```python
from build123d import *

# Parameters (mm, degrees)
BOSS_EXTRUDE1_DEPTH          = 5
BOSS_EXTRUDE1_DEPTH_BACK     = 7.5
SKETCH2_W                    = 57.31
SKETCH2_H                    = 43.46
SKETCH2_W_2                  = 53.31
SKETCH2_H_2                  = 39.46
FILLET1_R                    = 5
SKETCH3_R                    = 1
BOSS_EXTRUDE2_DEPTH          = 3
CUT_EXTRUDE1_DEPTH           = 2
CUT_EXTRUDE1_DRAFT           = 3
SKETCH5_R                    = 1
CUT_EXTRUDE1_PROFILE_2_DEPTH = 2
CUT_EXTRUDE1_PROFILE_2_DRAFT = 3
CUT_EXTRUDE1_PROFILE_3_DEPTH = 2
CUT_EXTRUDE1_PROFILE_3_DRAFT = 3
FILLET2_R                    = 1
SKETCH6_W                    = 2
SKETCH6_H                    = 40
BOSS_EXTRUDE3_DEPTH          = 2
FILLET3_R                    = 1


with BuildPart() as part:
    # Sketch2 → Boss-Extrude1 (new, two sides: drawn at the far end of the back side and taken through both)
    with BuildSketch(Plane(origin=(0, 0, 0), x_dir=(1, 0, 0), z_dir=(0, 1, 0)).offset(-BOSS_EXTRUDE1_DEPTH_BACK)):
        with Locations((-3, -1.5)):
            Rectangle(SKETCH2_W, SKETCH2_H)
        with Locations((-3, -1.5)):
            Rectangle(SKETCH2_W_2, SKETCH2_H_2, mode=Mode.SUBTRACT)
    extrude(amount=BOSS_EXTRUDE1_DEPTH + BOSS_EXTRUDE1_DEPTH_BACK)

    # Fillet1
    fillet1_edges = [part.edges().sort_by_distance(p)[0] for p in [
        (-29.655, -1.25, 21.23),
        (-29.655, -1.25, -18.23),
        (23.655, -1.25, -18.23),
        (23.655, -1.25, 21.23),
        (-31.655, -1.25, -20.23),
        (25.655, -1.25, -20.23),
        (25.655, -1.25, 23.23),
        (-31.655, -1.25, 23.23),
    ]]
    fillet(fillet1_edges, radius=FILLET1_R)

    # Sketch3 → Boss-Extrude2 (add)
    with BuildSketch(Plane.XZ.offset(7.5)):
        with BuildLine():
            Line((-31.655, 18.23), (-31.655, -15.23))
            ThreePointArc((-31.655, -15.23), (-30.190533906, -18.765533906), (-26.655, -20.23))
            Line((-26.655, -20.23), (20.655, -20.23))
            ThreePointArc((20.655, -20.23), (24.190533906, -18.765533906), (25.655, -15.23))
            Line((25.655, -15.23), (25.655, 18.23))
            ThreePointArc((25.655, 18.23), (24.190533906, 21.765533906), (20.655, 23.23))
            Line((20.655, 23.23), (-26.655, 23.23))
            ThreePointArc((-26.655, 23.23), (-30.190533906, 21.765533906), (-31.655, 18.23))
        make_face()
        with Locations(Location((-18.155, 11.5, 0), (0, 0, 270))):
            Circle(SKETCH3_R, mode=Mode.SUBTRACT)
        with Locations(Location((17.845, 11.5, 0), (0, 0, 270))):
            Circle(SKETCH3_R, mode=Mode.SUBTRACT)
        with Locations(Location((17.845, -12.5, 0), (0, 0, 270))):
            Circle(SKETCH3_R, mode=Mode.SUBTRACT)
    extrude(amount=BOSS_EXTRUDE2_DEPTH)


with BuildPart() as cut_extrude1_tool:
    # Sketch5 → Cut-Extrude1 (with draft: the straight prism first)
    with BuildSketch(Plane.XZ.offset(10.5)):
        Polygon((-18.155, 13.924871131), (-20.255, 12.712435565), (-20.255, 10.287564435), (-18.155, 9.075128869), (-16.055, 10.287564435), (-16.055, 12.712435565), align=None)
    extrude(amount=-CUT_EXTRUDE1_DEPTH)
    # Cut-Extrude1: the draft: its side faces are tilted about the plane it starts from
    cut_extrude1_sides = [cut_extrude1_tool.faces().sort_by_distance(p)[0] for p in [
        (-19.205, -9.5, 13.318653348),
        (-20.255, -9.5, 11.5),
        (-19.205, -9.5, 9.681346652),
        (-17.105, -9.5, 9.681346652),
        (-16.055, -9.5, 11.5),
        (-17.105, -9.5, 13.318653348),
    ]]
    draft(cut_extrude1_sides, Plane.XZ.offset(10.5), CUT_EXTRUDE1_DRAFT)


with BuildPart() as part_1:
    add(part.part)

    # Cut-Extrude1: cut by cut_extrude1_tool
    add(cut_extrude1_tool.part, mode=Mode.SUBTRACT)


with BuildPart() as cut_extrude1_profile_2_tool:
    # Sketch5 → Cut-Extrude1 profile 2 (with draft: the straight prism first)
    with BuildSketch(Plane.XZ.offset(10.5)):
        Polygon((17.857823878, 13.905392128), (15.745, 12.685552694), (15.745, 10.275489302), (17.857823878, 9.055649867), (19.945, 10.260681563), (19.945, 12.700360432), align=None)
        with Locations(Location((17.845, 11.5, 0), (0, 0, 270))):
            Circle(SKETCH5_R, mode=Mode.SUBTRACT)
    extrude(amount=-CUT_EXTRUDE1_PROFILE_2_DEPTH)
    # Cut-Extrude1 profile 2: the draft: its side faces are tilted about the plane it starts from
    cut_extrude1_profile_2_sides = [cut_extrude1_profile_2_tool.faces().sort_by_distance(p)[0] for p in [
        (16.801411939, -9.5, 13.295472411),
        (15.745, -9.5, 11.480520998),
        (16.801411939, -9.5, 9.665569584),
        (18.901411939, -9.5, 9.658165715),
        (19.945, -9.5, 11.480520998),
        (18.901411939, -9.5, 13.30287628),
        (17.845, -9.5, 12.5),
    ]]
    draft(cut_extrude1_profile_2_sides, Plane.XZ.offset(10.5), CUT_EXTRUDE1_PROFILE_2_DRAFT)


with BuildPart() as part_2:
    add(part_1.part)

    # Cut-Extrude1 profile 2: cut by cut_extrude1_profile_2_tool
    add(cut_extrude1_profile_2_tool.part, mode=Mode.SUBTRACT)


with BuildPart() as cut_extrude1_profile_3_tool:
    # Sketch5 → Cut-Extrude1 profile 3 (with draft: the straight prism first)
    with BuildSketch(Plane.XZ.offset(10.5)):
        Polygon((17.833837254, -10.086917044), (15.733837254, -11.299352609), (15.733837254, -13.724223739), (17.833837254, -14.936659305), (19.933837254, -13.724223739), (19.933837254, -11.299352609), align=None)
        with Locations(Location((17.845, -12.5, 0), (0, 0, 270))):
            Circle(SKETCH5_R, mode=Mode.SUBTRACT)
    extrude(amount=-CUT_EXTRUDE1_PROFILE_3_DEPTH)
    # Cut-Extrude1 profile 3: the draft: its side faces are tilted about the plane it starts from
    cut_extrude1_profile_3_sides = [cut_extrude1_profile_3_tool.faces().sort_by_distance(p)[0] for p in [
        (16.783837254, -9.5, -10.693134826),
        (15.733837254, -9.5, -12.511788174),
        (16.783837254, -9.5, -14.330441522),
        (18.883837254, -9.5, -14.330441522),
        (19.933837254, -9.5, -12.511788174),
        (18.883837254, -9.5, -10.693134826),
        (17.845, -9.5, -11.5),
    ]]
    draft(cut_extrude1_profile_3_sides, Plane.XZ.offset(10.5), CUT_EXTRUDE1_PROFILE_3_DRAFT)


with BuildPart() as part_3:
    add(part_2.part)

    # Cut-Extrude1 profile 3: cut by cut_extrude1_profile_3_tool
    add(cut_extrude1_profile_3_tool.part, mode=Mode.SUBTRACT)

    # Fillet2
    fillet2_edges = [part_3.edges().sort_by_distance(p)[0] for p in [
        (-3, 5, 21.23),
        (-29.655, 5, 1.5),
        (-3, 5, -18.23),
        (23.655, 5, 1.5),
        (-3, -7.5, -18.23),
        (-29.655, -7.5, 1.5),
        (-3, -7.5, 21.23),
        (23.655, -7.5, 1.5),
        (22.190533906, 5, 19.765533906),
        (22.190533906, -7.5, 19.765533906),
        (-28.190533906, 5, 19.765533906),
        (-28.190533906, -7.5, 19.765533906),
        (22.190533906, 5, -16.765533906),
        (22.190533906, -7.5, -16.765533906),
        (-28.190533906, 5, -16.765533906),
        (-28.190533906, -7.5, -16.765533906),
    ]]
    fillet(fillet2_edges, radius=FILLET2_R)

    # Sketch6 → Boss-Extrude3 (add, symmetric)
    # profile 1 of 2: a face of its own
    with BuildSketch(Plane(origin=(0, 0, 0), x_dir=(1, 0, 0), z_dir=(0, 1, 0))):
        with BuildLine():
            Line((-37.655, 20.23), (-37.655, -23.23))
            Line((-37.655, -23.23), (-26.655, -23.23))
            ThreePointArc((-26.655, -23.23), (-30.190533906, -21.765533906), (-31.655, -18.23))
            Line((-31.655, -18.23), (-31.655, 15.23))
            ThreePointArc((-31.655, 15.23), (-30.190533906, 18.765533906), (-26.655, 20.23))
            Line((-26.655, 20.23), (-37.655, 20.23))
        make_face()
        with Locations((-34.655, -1.77)):
            Rectangle(SKETCH6_W, SKETCH6_H, mode=Mode.SUBTRACT)
    # profile 2 of 2: a face of its own
    with BuildSketch(Plane(origin=(0, 0, 0), x_dir=(1, 0, 0), z_dir=(0, 1, 0))):
        with BuildLine():
            Line((20.655, 20.23), (31.655, 20.23))
            Line((31.655, 20.23), (31.655, -23.23))
            Line((31.655, -23.23), (20.655, -23.23))
            ThreePointArc((20.655, -23.23), (24.190533906, -21.765533906), (25.655, -18.23))
            Line((25.655, -18.23), (25.655, 15.23))
            ThreePointArc((25.655, 15.23), (24.190533906, 18.765533906), (20.655, 20.23))
        make_face()
        with Locations((28.655, -1.77)):
            Rectangle(SKETCH6_W, SKETCH6_H, mode=Mode.SUBTRACT)
    extrude(amount=BOSS_EXTRUDE3_DEPTH, both=True)

    # Fillet3
    fillet3_edges = [part_3.edges().sort_by_distance(p)[0] for p in [
        (-30.190533906, -10.5, 21.765533906),
        (-31.655, -10.5, 1.5),
        (-30.190533906, -10.5, -18.765533906),
        (-3, -10.5, -20.23),
        (24.190533906, -10.5, -18.765533906),
        (25.655, -10.5, 1.5),
        (24.190533906, -10.5, 21.765533906),
        (-3, -10.5, 23.23),
    ]]
    fillet(fillet3_edges, radius=FILLET3_R)


solid = part_3.part
```
Check sheet for the modelled part. Datum: model origin and axes. Units: mm. A direction names the side the tool comes from. Round coordinates to 2 decimals unless told otherwise and drop trailing zeros. Loops run counter-clockwise (first coordinate to the right, second up) from the corner with the lowest first, then second, coordinate; pieces in that order, holes last. Notation, with made-up numbers: M 36.5,41.5 L 62.5,41.5 A20 ccw 62.5,68.5 Z; hole C 60,-21.75 d7. An arc over 180 degrees is marked long. Answer as a JSON object with one key per item and string values.
1. Section check B-B (y = -4.75). Record the boundary of the cut face in (x, z) (3 decimals), plus the area to 3 significant figures.
Reply:
{"outline": "M -31.655,-15.23 A5 ccw -26.655,-20.23 L 20.655,-20.23 A5 ccw 25.655,-15.23 L 25.655,18.23 A5 ccw 20.655,23.23 L -26.655,23.23 A5 ccw -31.655,18.23 Z; hole M -29.655,-13.23 A5 ccw -24.655,-18.23 L 18.655,-18.23 A5 ccw 23.655,-13.23 L 23.655,16.23 A5 ccw 18.655,21.23 L -24.655,21.23 A5 ccw -29.655,16.23 Z", "area": "387 mm²"}
2. Section check A-A (z = -1). State how many separate pieces and enclosed holes the cut face has, plus the area to 3 significant figures.
Reply:
{"separate pieces": "3", "enclosed holes": "0", "area": "254 mm²"}
3. Gauge pin test, flat ends, axial feed: P1, Ø2, axis at x = 24, y = -3.5, coming from the -Z side; P2, Ø6, axis at y = -5.5, z = -2.5, coming from the +X side (3 decimals); P3, Ø1.5, axis at y = 3, z = 9.5, coming from the -X side (3 decimals). Record the tip position at first contact, or that the pin passes through.
Reply:
{"P1": "stops at z = -19.65", "P2": "stops at x = 25.655", "P3": "stops at x = -31.655"}
4. Section check C-C (y = -0.75). Record the boundary of the cut face in (x, z) (3 decimals), plus the area to 3 significant figures.
Reply:
{"outline": "M -37.655,-20.23 L 31.655,-20.23 L 31.655,23.23 L -37.655,23.23 Z; hole M -35.655,-18.23 L -33.655,-18.23 L -33.655,21.77 L -35.655,21.77 Z; hole M -29.655,-13.23 A5 ccw -24.655,-18.23 L 18.655,-18.23 A5 ccw 23.655,-13.23 L 23.655,16.23 A5 ccw 18.655,21.23 L -24.655,21.23 A5 ccw -29.655,16.23 Z; hole M 27.655,-18.23 L 29.655,-18.23 L 29.655,21.77 L 27.655,21.77 Z", "area": "770 mm²"}
5. Mould release check, pull along Y, two halves, no side actions. Record for faces 5 (the flat face through (18.93, -9.51, -10.66)), 6 (the flat face through (-33, 2, 1)), 7 (the flat face through (-35, 0, -18.23)): pulls with the +Y half, pulls with the -Y half, needs draft (parallel to the pull), parting line crosses it, or undercut.
Reply:
{"face 5": "undercut", "face 6": "pulls with the +Y half", "face 7": "needs draft"}
6. Scan lines: line 1 (X direction, y = -8.2, z = 11.5) (3 decimals); line 2 (X direction, y = -1.75, z = 0.5) (3 decimals); line 3 (X direction, y = -7.75, z = -12.5) (3 decimals). Record each from-to range of solid material in increasing order.
Reply:
{"line 1": "x = -31.655 to -19.155, -17.155 to 16.845, 18.845 to 25.655", "line 2": "x = -37.655 to -35.655, -33.655 to -29.655, 23.655 to 27.655, 29.655 to 31.655", "line 3": "x = -31.655 to 16.845, 18.845 to 25.655"}
7. Access from +Z, -Z, +X, -X, +Y, -Y to the whole of each face (thin tool, end or side, straight path). Record for faces 1 (the flat face through (29, 0, 21.77)), 2 (the flat face through (25.655, 4, 1)), 3 (the flat face through (-3, -1, -18.23)), 4 (the flat face through (-16.003, -9.514, 11.482)).
Reply:
{"face 1": "+Y, -Y", "face 2": "+Z, -Z, +X, +Y", "face 3": "+Y", "face 4": "none"}
